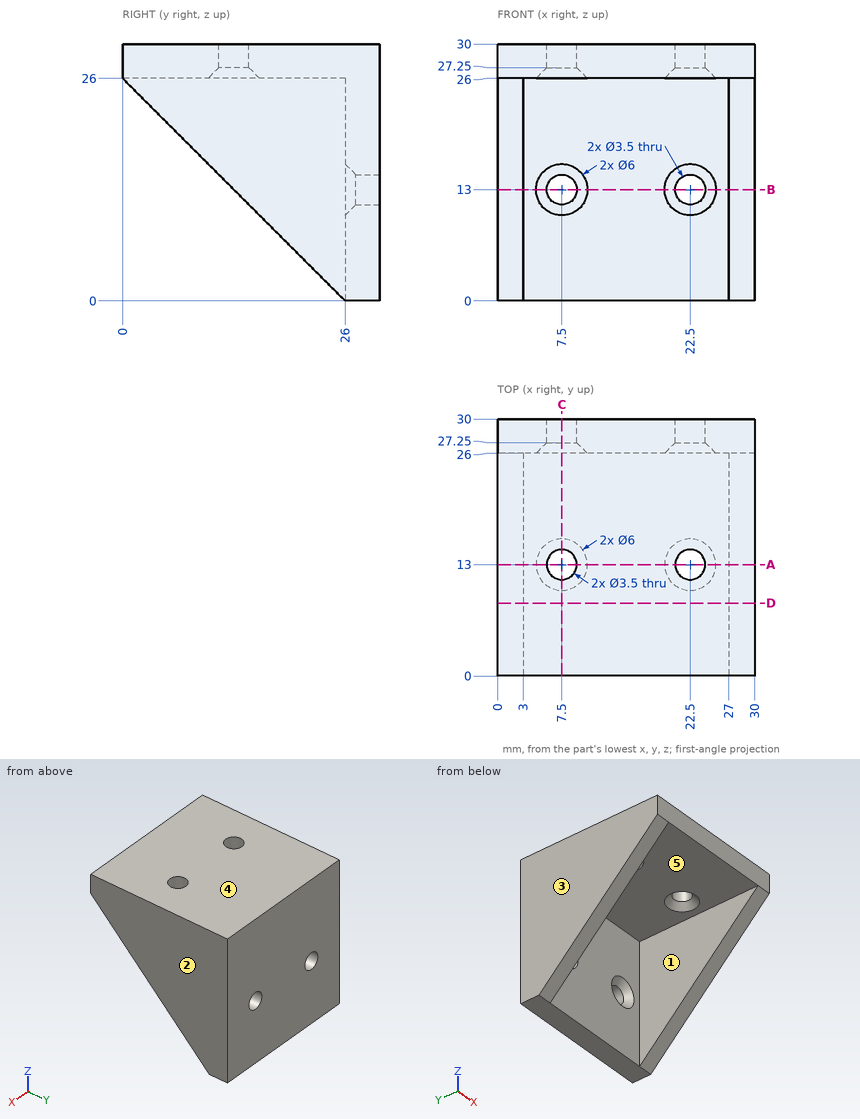
Geometry check sheet. Reference: drawing and pictorial views, mm from the part's lowest x, y, z. A direction names the side the tool comes from. Round coordinates to 2 decimals unless told otherwise and drop trailing zeros. Loops run counter-clockwise (first coordinate to the right, second up) from the corner with the lowest first, then second, coordinate; pieces in that order, holes last. Notation, with made-up numbers: (-12, 49.25) -> (5, 49.25) arc R29 cw to (5, 79.25) -> close; hole circle Ø10 at (-4, -15). An arc over 180 degrees is marked (long way). Answer as a JSON object with one key per item and string values.
Q1. Section check C-C (x = 7.5). Record the boundary of the cut face in (y, z), then the cut area to 3 significant figures.
Data:
{"outline": "(0, 26) -> (10, 26) -> (11.25, 27.25) -> (11.25, 30) -> (0, 30) -> close; (14.75, 27.25) -> (16, 26) -> (26, 26) -> (26, 16) -> (27.25, 14.75) -> (30, 14.75) -> (30, 30) -> (14.75, 30) -> close; (26, 0) -> (30, 0) -> (30, 11.25) -> (27.25, 11.25) -> (26, 10) -> close", "area": "193 mm2"}
Q2. Draft check along X on the marked faces 1, 2 and 3. Enter one of: pulls with the +X half, pulls with the -X half, needs draft (parallel to the pull), parting line crosses it, or undercut.
Data:
{"face 1": "undercut", "face 2": "pulls with the +X half", "face 3": "pulls with the -X half"}
Q3. Go/stop test with flat-tipped pins: P1, Ø7, axis at x = 19, y = 7.5, coming from the -Z side; P2, Ø10, axis at x = 24, z = 16.5, coming from the -Y side; P3, Ø7, axis at x = 18, z = 15, coming from the -Y side; P4, Ø2, axis at x = 7.5, z = 13, coming from the +Y side. Record where each tip stops, or that it passes through.
Data:
{"P1": "stops at z = 26", "P2": "stops at y = 5.5", "P3": "stops at y = 26", "P4": "passes through"}
Q4. Scan lines: line 1 (X direction, y = 13, z = 28); line 2 (Z direction, x = 22.5, y = 28.75). Record each from-to range of solid material in increasing order. Write a range as from..to.
Data:
{"line 1": "x = 0..5.75, 9.25..20.75, 24.25..30", "line 2": "z = 0..11.25, 14.75..30"}
Q5. Section check A-A (y = 13). Record the boundary of the cut face in (x, z), then the cut area to 3 significant figures.
Data:
{"outline": "(0, 13) -> (3, 13) -> (3, 26) -> (4.5, 26) -> (5.75, 27.25) -> (5.75, 30) -> (0, 30) -> close; (9.25, 27.25) -> (10.5, 26) -> (19.5, 26) -> (20.75, 27.25) -> (20.75, 30) -> (9.25, 30) -> close; (24.25, 27.25) -> (25.5, 26) -> (27, 26) -> (27, 13) -> (30, 13) -> (30, 30) -> (24.25, 30) -> close", "area": "167 mm2"}
Q6. Access from +Z, -Z, +X, -X, +Y, -Y to the whole of each face (thin tool, end or side, straight path). Record for the marked faces 4 and 5.
Data:
{"face 4": "+Z, +X, -X, +Y, -Y", "face 5": "-Z, -Y"}
Q7. Section check D-D (y = 8.5). Record the boundary of the cut face in (x, z).
Data:
{"outline": "(0, 17.5) -> (3, 17.5) -> (3, 26) -> (27, 26) -> (27, 17.5) -> (30, 17.5) -> (30, 30) -> (0, 30) -> close"}
